Design review of the part built by this model. Coordinates are the model's own, in mm. A direction names the side the tool comes from. Give positions to 0.01 mm unless a question says otherwise; leave off trailing zeros. Loops run counter-clockwise (first coordinate to the right, second up) from the corner with the lowest first, then second, coordinate; pieces in that order, holes last. Notation, with made-up numbers: M 69.25,31.25 L 94.25,31.25 A17 cw 94.25,40.25 Z; hole C 43.25,5.5 d5. An arc over 180 degrees is marked long. Use a Markdown table: item, result. Add a question column.
(1) Add section C-C, the plane z = -13.5. Give the boundary of the cut face in (x, y), then the cut area to 3 significant figures.
(2) Add section B-B, the plane y = 2. Give the boundary of the cut face in (x, z) (3 decimals), then the cut area to 3 significant figures.
(3) For probe 1 along Z at (x, y) = (10, 1.3) (3 decimals); probe 2 along X at (y, z) = (1.45, -10) (3 decimals); probe 3 along X at (y, z) = (3.75, -10), list the stretches that pass through material, from the lowest coordinate up.
(4) For faces 1 (the face through (-33.398, 1.972, 0.814)), 2 (the face through (7, 1, 40)), 3 (the face through (14.26, 3.51, 13.71)), list the 3-axis set-ups (+Z, -Z, +X, -X, +Y, -Y) from which the entire face can be reached by the end or side of a thin tool; tool diameter is ignored.
(5) Draft analysis for pull direction X (two halves, no side actions). For faces 4 (the face through (-27.74, 3.51, -7.29)), 5 (the face through (-40, 1, -8)), 6 (the face through (19.43, 1.48, -19.4)), state which applies: pulls with the +X half, pulls with the -X half, needs draft (parallel to the pull), parting line crosses it, or undercut.
(6) Add section A-A, the plane x = 10. State how many separate pieces and enclosed holes the cut face has, then the cut area to 3 significant figures.
(7) Insertion check: pin 1 Ø7 at (x, z) = (-11, -10) entering from +Y; pin 2 Ø1.5 at (y, z) = (2.5, 8.5) entering from -X; pin 3 Ø1.2 at (y, z) = (1, 23) entering from -X; pin 4 Ø6 at (x, z) = (-5.5, 24.5) entering from +Y (3 decimals). Each pin has a flat end and moves straight along its axis. Give the tip position at first contact, or say it passes through.
```python
from build123d import *

# Parameters (mm, degrees)
SKETCH1_R           = 2.625
BOSS_EXTRUDE1_DEPTH = 4
FILLET1_R           = 20
FILLET2_R           = 3
SKETCH2_R           = 5.05
CUT_EXTRUDE1_DEPTH  = 1
FILLET3_R           = 1


with BuildPart() as part:
    # Sketch1 → Boss-Extrude1 (new body)
    with BuildSketch(Plane(origin=(0, 0, 0), x_dir=(1, 0, 0), z_dir=(0, 1, 0))):
        with BuildLine():
            Line((2, -40), (18, -40))
            ThreePointArc((18, -40), (19.414213562, -39.414213562), (20, -38))
            Line((20, -38), (20, -10.175438596))
            Line((20, -10.175438596), (20, 18))
            ThreePointArc((20, 18), (19.414213562, 19.414213562), (18, 20))
            Line((18, 20), (-38, 20))
            ThreePointArc((-38, 20), (-39.414213562, 19.414213562), (-40, 18))
            Line((-40, 18), (-40, 2))
            Line((-40, 2), (-40, -4))
            Line((-40, -4), (-4, -40))
            Line((-4, -40), (2, -40))
        make_face()
        with Locations(Location((-32, 10, 0), (0, 0, 270))):
            Circle(SKETCH1_R, mode=Mode.SUBTRACT)
        with Locations(Location((-11, 10, 0), (0, 0, 270))):
            Circle(SKETCH1_R, mode=Mode.SUBTRACT)
        with Locations(Location((10, -32, 0), (0, 0, 270))):
            Circle(SKETCH1_R, mode=Mode.SUBTRACT)
        with Locations(Location((10, 10, 0), (0, 0, 270))):
            Circle(SKETCH1_R, mode=Mode.SUBTRACT)
        with Locations(Location((10, -11, 0), (0, 0, 270))):
            Circle(SKETCH1_R, mode=Mode.SUBTRACT)
        Polygon((0, 0), (0, -34.343145751), (-4, -34.343145751), (-34.343145751, -4), (-34.343145751, 0), align=None, mode=Mode.SUBTRACT)
    extrude(amount=BOSS_EXTRUDE1_DEPTH)

    # Fillet1
    fillet1_edges = [part.edges().sort_by_distance(p)[0] for p in [
        (0, 2, 0),
    ]]
    fillet(fillet1_edges, radius=FILLET1_R)

    # Fillet2
    # the kernel refuses this fillet: 3 mm, written as the material it adds along each edge
    with BuildSketch(Plane(origin=(-4, 0, 34.343145751), x_dir=(1, 0, 0), z_dir=(0, 1, 0)), Plane(origin=(-34.343145751, 0, 4), x_dir=(0.7071067811865454, 0, 0.7071067811865497), z_dir=(0, 1, 0))) as fillet2_piece_1:
        with BuildLine():
            CenterArc((FILLET2_R * 0.414213562373, FILLET2_R), FILLET2_R, 225, 45)
            Line((-FILLET2_R * 0.292893218813, FILLET2_R * 0.292893218813), (0, 0))
            Line((0, 0), (FILLET2_R * 0.414213562373, 0))
        make_face()
    extrude(amount=4)
    with BuildSketch(Plane(origin=(0, 0, 34.343145751), x_dir=(0, 0, -1), z_dir=(0, 1, 0))) as fillet2_piece_2:
        with BuildLine():
            CenterArc((FILLET2_R, FILLET2_R), FILLET2_R, 180, 90)
            Line((0, FILLET2_R), (0, 0))
            Line((0, 0), (FILLET2_R, 0))
        make_face()
    extrude(amount=4)
    with BuildSketch(Plane(origin=(-34.343145751, 0, 0), x_dir=(1, 0, 0), z_dir=(0, 1, 0))) as fillet2_piece_3:
        with BuildLine():
            CenterArc((FILLET2_R, -FILLET2_R), FILLET2_R, 90, 90)
            Line((0, -FILLET2_R), (0, 0))
            Line((0, 0), (FILLET2_R, 0))
        make_face()
    extrude(amount=4)
    # the kernel refuses this fillet: 3 mm, written as the material it takes off along each edge
    with BuildSketch(Plane(origin=(-40, -3.106601718, 4), x_dir=(0, 0, -1), z_dir=(0, 1, 0))) as fillet2_2_piece_1:
        with BuildLine():
            CenterArc((FILLET2_R * 0.414213562373, -FILLET2_R), FILLET2_R, 90, 45)
            Line((-FILLET2_R * 0.292893218813, -FILLET2_R * 0.292893218813), (0, 0))
            Line((0, 0), (FILLET2_R * 0.414213562373, 0))
        make_face()
    extrude(amount=10.213203436, mode=Mode.SUBTRACT)
    with BuildSketch(Plane(origin=(-4, -3.106601718, 40), x_dir=(1, 0, 0), z_dir=(0, 1, 0))) as fillet2_2_piece_2:
        with BuildLine():
            CenterArc((FILLET2_R * 0.414213562373, FILLET2_R), FILLET2_R, 225, 45)
            Line((-FILLET2_R * 0.292893218813, FILLET2_R * 0.292893218813), (0, 0))
            Line((0, 0), (FILLET2_R * 0.414213562373, 0))
        make_face()
    extrude(amount=10.213203436, mode=Mode.SUBTRACT)

    # Sketch2 → Cut-Extrude1 (cut)
    with BuildSketch(Plane(origin=(0, 4, 0), x_dir=(1, 0, 0), z_dir=(0, 1, 0))):
        with Locations(Location((-32, 10, 0), (0, 0, 270))):
            Circle(SKETCH2_R)
        with Locations(Location((-11, 10, 0), (0, 0, 270))):
            Circle(SKETCH2_R)
        with Locations(Location((10, 10, 0), (0, 0, 270))):
            Circle(SKETCH2_R)
        with Locations(Location((10, -11, 0), (0, 0, 270))):
            Circle(SKETCH2_R)
        with Locations(Location((10, -32, 0), (0, 0, 270))):
            Circle(SKETCH2_R)
    extrude(amount=-CUT_EXTRUDE1_DEPTH, mode=Mode.SUBTRACT)

    # Fillet3
    fillet3_edges = [part.edges().sort_by_distance(p)[0] for p in [
        (-10, 4, -20),
        (-39.414213562, 4, -19.414213562),
        (-40, 4, -7.621320344),
        (19.414213562, 4, 39.414213562),
        (20, 4, 10),
        (-22, 4, 22),
        (7.621320344, 4, 40),
        (-3.90540961, 4, 39.771638598),
        (-39.771638598, 4, 3.90540961),
        (19.414213562, 4, -19.414213562),
    ]]
    fillet(fillet3_edges, radius=FILLET3_R)


solid = part.part
```
Established:
| question | item | result |
|---|---|---|
| 1 | outline | M -40,0 L 20,0 L 20,3 A1 ccw 19,4 L 13.64,4 L 13.64,3 L 6.36,3 L 6.36,4 L -7.36,4 L -7.36,3 L -14.64,3 L -14.64,4 L -28.36,4 L -28.36,3 L -35.64,3 L -35.64,4 L -39,4 A1 ccw -40,3 Z |
| 1 | area | 218 mm^2 |
| 2 | outline | M -40,-18 A2 ccw -38,-20 L 18,-20 A2 ccw 20,-18 L 20,38 A2 ccw 18,40 L -2.757,40 A3 ccw -4.879,39.121 L -39.121,4.879 A3 ccw -40,2.757 Z; hole C -32,-10 d5.25; hole M -34.341,2.879 A3 ccw -31.343,0 L -20,0 A20 ccw 0,20 L 0,31.343 A3 ccw -2.879,34.341 A3 ccw -4.879,33.464 L -33.464,4.879 A3 ccw Z; hole C -11,-10 d5.25; hole C 10,-10 d5.25; hole C 10,11 d5.25; hole C 10,32 d5.25 |
| 2 | area | 2,210 mm^2 |
| 3 | probe 1 | -20 to -12.625, -7.375 to 8.375, 13.625 to 29.375, 34.625 to 40 |
| 3 | probe 2 | -40 to -34.625, -29.375 to -13.625, -8.375 to 7.375, 12.625 to 20 |
| 3 | probe 3 | -39.66 to -37.05, -26.95 to -16.05, -5.95 to 4.95, 15.05 to 19.66 |
| 4 | face 1 | +Y, -Y |
| 4 | face 2 | +Z, +X, -X, +Y, -Y |
| 4 | face 3 | +Y |
| 5 | face 4 | undercut |
| 5 | face 5 | pulls with the -X half |
| 5 | face 6 | pulls with the +X half |
| 6 | separate pieces | 4 |
| 6 | enclosed holes | 0 |
| 6 | area | 162 mm^2 |
| 7 | pin 1 | y = 3 |
| 7 | pin 2 | x = -36.25 |
| 7 | pin 3 | x = -21.6 |
| 7 | pin 4 | through |
